Read the model definition and answer for the solid it produces. Units are mm, in the model's axes. A direction names the side the tool comes from. Coordinates: 2 decimals unless noted, no trailing zeros. Loops run counter-clockwise (first coordinate to the right, second up) from the corner with the lowest first, then second, coordinate; pieces in that order, holes last. Notation, with made-up numbers: (7.25, 81) -> (13.25, 81) arc R21 cw to (13.25, 119) -> close; hole circle Ø5 at (52, -37). An arc over 180 degrees is marked (long way). Answer as CSV lines item,"result".
```python
from build123d import *

# Parameters (mm, degrees)
SKETCH1_W           = 6.7846
SKETCH1_H           = 5.0066
SKETCH1_W_2         = 3.8846
SKETCH1_H_2         = 2.1066
BOSS_EXTRUDE1_DEPTH = 2.3
SKETCH2_W           = 7.3
SKETCH2_H           = 7.3
BOSS_EXTRUDE2_DEPTH = 2.5
CHAMFER1_SIZE       = 1
SKETCH3_W           = 3.8846
SKETCH3_H           = 2.1066
CUT_EXTRUDE1_DEPTH  = 1.1


with BuildPart() as part:
    # Sketch1 → Boss-Extrude1 (new body)
    with BuildSketch(Plane.XY):
        Rectangle(SKETCH1_W, SKETCH1_H)
        Rectangle(SKETCH1_W_2, SKETCH1_H_2, mode=Mode.SUBTRACT)
    extrude(amount=-BOSS_EXTRUDE1_DEPTH)

    # Sketch2 → Boss-Extrude2 (add)
    with BuildSketch(Plane.XY):
        Rectangle(SKETCH2_W, SKETCH2_H)
    extrude(amount=BOSS_EXTRUDE2_DEPTH)

    # Chamfer1
    chamfer1_edges = [part.edges().sort_by_distance(p)[0] for p in [
        (3.65, -3.65, 1.25),
        (3.65, 3.65, 1.25),
        (-3.65, 3.65, 1.25),
        (-3.65, -3.65, 1.25),
        (3.65, 0, 2.5),
        (0, 3.65, 2.5),
        (-3.65, 0, 2.5),
        (0, -3.65, 2.5),
    ]]
    chamfer(chamfer1_edges, length=CHAMFER1_SIZE)

    # Sketch3 → Cut-Extrude1 (cut)
    with BuildSketch(Plane(origin=(0, 0, 0), x_dir=(-1, 0, 0), z_dir=(0, 0, -1))):
        Rectangle(SKETCH3_W, SKETCH3_H)
    extrude(amount=-CUT_EXTRUDE1_DEPTH, mode=Mode.SUBTRACT)


solid = part.part
```
Q1. For a pull along X with two mould halves and no side action, classify faces 1 (the face through (3.65, 0, 1)), 2 (the face through (-1.942, 0, -1)), 3 (the face through (0, 3, 0)) as pulls with the +X half, pulls with the -X half, needs draft (parallel to the pull), parting line crosses it, or undercut.
Results:
face 1,"pulls with the +X half"
face 2,"undercut"
face 3,"needs draft"
Q2. Find the intervals of material crossed by probe 1 along Y at (x, z) = (1.75, 0.7); probe 2 along Y at (x, z) = (0.25, -0.85); probe 3 along X at (y, z) = (-0.75, 0.8), in increasing order. Write a range as [from, to].
Results:
probe 1,"y = [-3.65, -1.05], [1.05, 3.65]"
probe 2,"y = [-2.5, -1.05], [1.05, 2.5]"
probe 3,"x = [-3.65, -1.94], [1.94, 3.65]"
Q3. A cutting plane is placed at C-C, the plane y = -1.75. Write down the section's boundary in (x, z), and give its area (3 significant figures).
Results:
outline,"(-3.65, 0) -> (-3.39, 0) -> (-3.39, -2.3) -> (3.39, -2.3) -> (3.39, 0) -> (3.65, 0) -> (3.65, 1.5) -> (2.65, 2.5) -> (-2.65, 2.5) -> (-3.65, 1.5) -> close"
area,"32.9 mm²"
Q4. A cutting plane is placed at B-B, the plane z = -1.7. Write down the section's boundary in (x, y).
Results:
outline,"(-3.39, -2.5) -> (3.39, -2.5) -> (3.39, 2.5) -> (-3.39, 2.5) -> close; hole (-1.94, -1.05) -> (1.94, -1.05) -> (1.94, 1.05) -> (-1.94, 1.05) -> close"
Q5. Given pin 1 Ø0.7 at (y, z) = (1, -1.5) entering from +X; pin 2 Ø0.6 at (y, z) = (0, -1.5) entering from -X; pin 3 Ø0.7 at (x, z) = (1.5, -0.5) entering from +Y, each flat-ended and moving along its own axis, determine where each tip first touches the part or whether it passes through.
Results:
pin 1,"stops at x = 3.39"
pin 2,"stops at x = -3.39"
pin 3,"stops at y = 2.5"
Q6. A cutting plane is placed at A-A, the plane x = -2.75. Write down the section's boundary in (y, z).
Results:
outline,"(-3.55, 0) -> (-2.5, 0) -> (-2.5, -2.3) -> (2.5, -2.3) -> (2.5, 0) -> (3.55, 0) -> (3.55, 1.5) -> (2.65, 2.4) -> (-2.65, 2.4) -> (-3.55, 1.5) -> close"
Q7. A cutting plane is placed at D-D, the plane z = 1.65. Write down the section's boundary in (x, y).
Results:
outline,"(-3.5, -2.65) -> (-2.65, -3.5) -> (2.65, -3.5) -> (3.5, -2.65) -> (3.5, 2.65) -> (2.65, 3.5) -> (-2.65, 3.5) -> (-3.5, 2.65) -> close"
Q8. For faces 4 (the face through (0, -1.053, -1)), 5 (the face through (0, 2.503, -1)), 6 (the face through (-3.392, 0, -1)), determine the directions among +Z, -Z, +X, -X, +Y, -Y from which every point of the face is accessible in a straight line to the end or side of a thin tool.
Results:
face 4,"-Z"
face 5,"-Z, +X, -X, +Y"
face 6,"-Z, -X, +Y, -Y"
